Could you check a few things on this model? Use its own coordinates, in mm. Face numbers are marked on the shaded views. A direction names the side the tool comes from. Round coordinates to 2 decimals unless told otherwise and drop trailing zeros. Order: outer loops, then holes, each group sorted by start corner. A loop starts at its lowest first (then second) coordinate and runs counter-clockwise, first axis right, second up. Notation, with made-up numbers: (48.5, 6) - (106.5, 6) arc R19 ccw to (106.5, 34) - close; hole circle Ø9 at (21.25, -19). An arc over 180 degrees is marked (long way). Use one line per item in the form item = value.
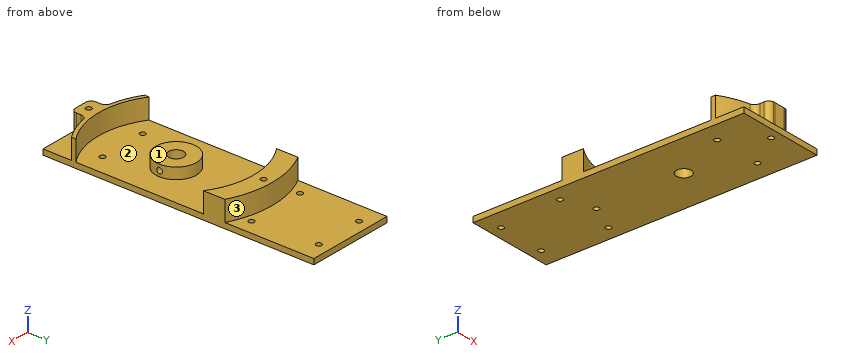
from build123d import *

# Parameters (mm, degrees)
SKETCH1_W                = 47.380920583
SKETCH1_H                = 3
BOSS_EXTRUDE2_DEPTH      = 32.13354
BOSS_EXTRUDE2_DEPTH_BACK = 115
SKETCH3_R                = 1.5
SKETCH3_R_2              = 4
CUT_EXTRUDE1_DEPTH       = 10
SKETCH4_R                = 1.5
BOSS_EXTRUDE6_DEPTH      = 11
SKETCH4_3_R              = 1.5
CUT_EXTRUDE2_DEPTH       = 10
SKETCH3_5_R              = 11
SKETCH3_5_R_2            = 4
BOSS_EXTRUDE7_DEPTH      = 9
SKETCH8_R                = 1.5
CUT_EXTRUDE3_DEPTH       = 9


with BuildPart() as part:
    # Sketch1 → Boss-Extrude2 (new body, two sides)
    with BuildSketch(Plane(origin=(0, 0, 0), x_dir=(1, 0, 0), z_dir=(0, 1, 0))) as boss_extrude2_sk:
        with Locations((-0.010103172, -96.309011723)):
            Rectangle(SKETCH1_W, SKETCH1_H)
    extrude(amount=BOSS_EXTRUDE2_DEPTH)
    extrude(boss_extrude2_sk.sketch, amount=-BOSS_EXTRUDE2_DEPTH_BACK)

    # Sketch3 → Cut-Extrude1 (cut)
    with BuildSketch(Plane(origin=(0, 0, 94.809011723), x_dir=(-1, 0, 0), z_dir=(0, 0, -1))):
        with Locations((-12.989896828, -91.59646)):
            Circle(SKETCH3_R)
        with Locations((0.010103172, -62.5)):
            Circle(SKETCH3_R_2)
        with Locations((13.010103172, -91.59646)):
            Circle(SKETCH3_R)
        with Locations((-15.690228452, -8.417274823)):
            Circle(SKETCH3_R)
        with Locations((15.713451538, -8.447491658)):
            Circle(SKETCH3_R)
        with Locations((13.010103172, 25.86354)):
            Circle(SKETCH3_R)
        with Locations((-12.989896828, 25.86354)):
            Circle(SKETCH3_R)
    extrude(amount=-CUT_EXTRUDE1_DEPTH, mode=Mode.SUBTRACT)

    # Sketch4 → Boss-Extrude6 (add)
    with BuildSketch(Plane.XY.offset(97.809011723)):
        with BuildLine():
            ThreePointArc((8.69292522, -105.630700166), (16.466971046, -103.298358119), (23.68035712, -99.577784335))
            Line((23.68035712, -99.577784335), (23.68035712, -97.180860589))
            ThreePointArc((23.68035712, -97.180860589), (-0.010103172, -104.5), (-23.700563463, -97.180860589))
            Line((-23.700563463, -97.180860589), (-23.700563463, -99.577784335))
            ThreePointArc((-23.700563463, -99.577784335), (-16.487177389, -103.298358119), (-8.713131563, -105.630700166))
            ThreePointArc((-8.713131563, -105.630700166), (-0.010103172, -106.5), (8.69292522, -105.630700166))
        make_face()
        with BuildLine():
            ThreePointArc((-23.700563463, -27.819139411), (-0.010103172, -20.5), (23.68035712, -27.819139411))
            Line((23.68035712, -27.819139411), (23.68035712, -25.422215665))
            ThreePointArc((23.68035712, -25.422215665), (-0.010103172, -18.5), (-23.700563463, -25.422215665))
            Line((-23.700563463, -25.422215665), (-23.700563463, -27.819139411))
        make_face()
        with BuildLine():
            ThreePointArc((6.263230229, -109.027045372), (6.926559458, -106.93432478), (8.69292522, -105.630700166))
            ThreePointArc((8.69292522, -105.630700166), (-0.010103172, -106.5), (-8.713131563, -105.630700166))
            ThreePointArc((-8.713131563, -105.630700166), (-6.946765802, -106.93432478), (-6.283436573, -109.027045372))
            Line((-6.283436573, -109.027045372), (-6.283436573, -111.414142146))
            ThreePointArc((-6.283436573, -111.414142146), (-5.602096929, -113.317773977), (-3.867560473, -114.35672592))
            ThreePointArc((-3.867560473, -114.35672592), (-3.432425137, -114.387259634), (-2.997048979, -114.414142146))
            Line((-2.997048979, -114.414142146), (2.976842636, -114.414142146))
            ThreePointArc((2.976842636, -114.414142146), (3.412218794, -114.387259634), (3.84735413, -114.35672592))
            ThreePointArc((3.84735413, -114.35672592), (5.581890586, -113.317773977), (6.263230229, -111.414142146))
            Line((6.263230229, -111.414142146), (6.263230229, -109.027045372))
        make_face()
        with Locations((-0.010103172, -110)):
            Circle(SKETCH4_R, mode=Mode.SUBTRACT)
        with BuildLine():
            ThreePointArc((-23.700563463, -25.422215665), (-0.010103172, -18.5), (23.68035712, -25.422215665))
            Line((23.68035712, -25.422215665), (23.68035712, -16.210021698))
            ThreePointArc((23.68035712, -16.210021698), (-0.010103172, -10.5), (-23.700563463, -16.210021698))
            Line((-23.700563463, -16.210021698), (-23.700563463, -25.422215665))
        make_face()
        with Locations((-0.010103172, -15)):
            Circle(SKETCH4_R, mode=Mode.SUBTRACT)
    extrude(amount=BOSS_EXTRUDE6_DEPTH)

    # Sketch4_3 → Cut-Extrude2 (cut)
    with BuildSketch(Plane.XY.offset(97.809011723)):
        with Locations((-0.010103172, -110)):
            Circle(SKETCH4_3_R)
        with Locations((-0.010103172, -15)):
            Circle(SKETCH4_3_R)
    extrude(amount=-CUT_EXTRUDE2_DEPTH, mode=Mode.SUBTRACT)

    # Sketch3_5 → Boss-Extrude7 (add)
    with BuildSketch(Plane(origin=(0, 0, 94.809011723), x_dir=(-1, 0, 0), z_dir=(0, 0, -1))):
        with Locations((0.010103172, -62.5)):
            Circle(SKETCH3_5_R)
        with Locations((0.010103172, -62.5)):
            Circle(SKETCH3_5_R_2, mode=Mode.SUBTRACT)
    extrude(amount=-BOSS_EXTRUDE7_DEPTH)

    # Sketch8 → Cut-Extrude3 (cut)
    with BuildSketch(Plane(origin=(10.989896828, 0, 0), x_dir=(0, 0, -1), z_dir=(1, 0, 0))):
        with Locations((-100.78123084, -62.396797047)):
            Circle(SKETCH8_R)
    extrude(amount=-CUT_EXTRUDE3_DEPTH, mode=Mode.SUBTRACT)


solid = part.part
Item 1: Will these pins go through, and if not, where does the flat tip stop? P1, Ø2.5, axis at x = -15.71, y = -8.45, coming from the -Z side; P2, Ø5, axis at x = -13.01, y = 25.86, coming from the -Z side; P3, Ø14, axis at x = -0.5, y = -77.5, coming from the +Z side; P4, Ø5, axis at x = -1, z = 106.5, coming from the +Y side.
Found:
P1 = through
P2 = 94.81
P3 = 103.81
P4 = -10.5
Item 2: Imagine slicing it at B-B on z = 96.5. State how many separate pieces and enclosed holes the cut face has, plus the area to 3 significant figures.
Found:
separate_pieces = 1
enclosed_holes = 9
area = 6,860 mm2
Item 3: For the marked faces 1, 2 and 3, which set-ups out of +Z, -Z, +X, -X, +Y, -Y let a thin tool reach every point of the face, with its end or its side?
Found:
face_1 = +Z, +X, -X
face_2 = +Z
face_3 = +Z, +Y
Item 4: Imagine slicing it at C-C on y = -46.5. Please give me the cut outline in (x, z).
Found:
outline = (-23.7, 94.81) - (23.68, 94.81) - (23.68, 97.81) - (-23.7, 97.81) - close
Item 5: I need wall thicknesses on L1, parallel to X at y = -110, z = 105.5; L2, parallel to Z at x = 19, y = -86.5; L3, parallel to Y at x = -10.5, z = 108.25. Which ranges of each line are inside material? Lowest first, please.
Found:
L1 = -6.28 to -1.51, 1.49 to 6.26
L2 = 94.81 to 97.81
L3 = -105.23 to -103.17, -21.83 to -11.57
Item 6: Imagine slicing it at A-A on z = 105.5. Please give me the cut outline in (x, y), plus the area to 3 significant figures.
Found:
outline = (-23.7, -99.58) arc R44 ccw to (-8.71, -105.63) arc R3.55 cw to (-6.28, -109.03) - (-6.28, -111.41) arc R3 ccw to (-3.87, -114.36) arc R52 ccw to (-3, -114.41) - (2.98, -114.41) arc R52 ccw to (3.85, -114.36) arc R3 ccw to (6.26, -111.41) - (6.26, -109.03) arc R3.55 cw to (8.69, -105.63) arc R44 ccw to (23.68, -99.58) - (23.68, -97.18) arc R42 cw to (-23.7, -97.18) - close; (-23.7, -27.82) arc R42 cw to (23.68, -27.82) - (23.68, -16.21) arc R52 ccw to (-23.7, -16.21) - close; hole circle Ø3 at (-0.01, -110); hole circle Ø3 at (-0.01, -15)
area = 684 mm2
